Autodesk Inventor part; units mm, degrees
ref_plane "YZ Plane" through (0, 0, 0) normal (1, 0, 0) x (0, 1, 0)
ref_plane "XZ Plane" through (0, 0, 0) normal (0, 1, 0) x (-1, 0, 0)
ref_plane "XY Plane" through (0, 0, 0) normal (0, 0, 1) x (1, 0, 0)
sketch "Boceto1" plane through (0, 0, 0) normal (0, 1, 0) x (-1, 0, 0)
  line L0 (-10, 37.5) -> (10, 37.5)
  line L1 (10, 37.5) -> (10, -37.5)
  line L2 (10, -37.5) -> (-10, -37.5)
  line L3 (-10, -37.5) -> (-10, 37.5)
  line L4 (-10, 37.5) -> (10, -37.5) construction
  line L5 (10, 37.5) -> (-10, -37.5) construction
  circle A0 centre (0, -27.5) radius 8.125
  point P0 (0, 0)
  point P1 (5.4787, -34.25)
  point P2 (-5.4787, -34.25)
  dimension "d0" = 20
  dimension "d23" = 65
  dimension "d24" = 10
  dimension "d25" = 16.25
extrude "Extrusión1" add sketch "Boceto1" along normal blind 12 contours L0 L1 L2 L3 | A0
sketch "Boceto5" plane through (0, 12, 0) normal (0, 1, 0) x (1, 0, 0)
  circle A0 centre (0, 27.5) radius 8.125
  line L0 (10, 37.5) -> (-10, 37.5)
  line L1 (-10, -37.5) -> (10, -37.5)
  point P0 (0, 0)
  dimension "d26" = 16.25
  dimension "d36" = 65
extrude "Extrusión5" cut sketch "Boceto5" against normal blind 7
sketch "Boceto6" plane through (0, 5, -27.5) normal (0, 1, 0) x (1, 0, 0)
  circle A0 centre (0, 0) radius 6.5
  point P0 (0, -27.5)
  dimension "d30" = 13
extrude "Extrusión6" cut sketch "Boceto6" against normal through all
sketch "Boceto7" plane through (0, 12, 0) normal (0, 1, 0) x (1, 0, 0)
  circle A0 centre (0, 27.5) radius 8.125
  circle A1 centre (0, 27.5) radius 15
  point P0 (0, 0)
  dimension "d33" = 30
extrude "Extrusión7" cut sketch "Boceto7" against normal blind 2
fillet "Empalme5" radius 5 2 edges at (-10, 6, 37.5) (10, 6, 37.5)
fillet "Empalme6" radius 5 2 edges at (10, 5, -37.5) (-10, 5, -37.5)
sketch "Boceto8" plane through (0, 0, 0) normal (0, -1, 0) x (1, 0, 0)
  circle A0 centre (0, 31.5) radius 2.7
  circle A1 centre (0, 15.5) radius 2.7
  line L0 (-5, 37.5) -> (5, 37.5)
  circle A2 centre (0, -0.5) radius 2.7
  point P0 (0, 0)
  dimension "d39" = 5.4
  dimension "d40" = 6
  dimension "d41" = 16
  dimension "d47" = 16
extrude "Extrusión8" cut sketch "Boceto8" against normal through all
sketch "Boceto9" plane through (0, 0, 0) normal (0, -1, 0) x (1, 0, 0)
  circle A0 centre (0, 31.5) radius 2.7
  circle A1 centre (0, 31.5) radius 4.65
  circle A2 centre (0, 15.5) radius 2.7
  circle A3 centre (0, 15.5) radius 4.65
  circle A4 centre (0, -0.5) radius 2.7
  circle A5 centre (0, -0.5) radius 4.65
  point P0 (0, 0)
  dimension "d44" = 9.3
extrude "Extrusión9" cut sketch "Boceto9" against normal blind 2 contours A0 | A1 | A2 | A3 | A4 | A5
sketch "Boceto2" plane through (0, 12, 0) normal (0, 1, 0) x (1, 0, 0)
  line L0 (10, 37.5) -> (-10, 37.5)
  line L1 (-10, 37.5) -> (5, 37.5)
  line L2 (5, 37.5) -> (5, 77.5)
  line L3 (5, 77.5) -> (-5, 77.5)
  line L4 (-5, 77.5) -> (-5, 37.5)
  circle A0 centre (0, 70) radius 2.7
  line L5 (10, -37.5) -> (10, 37.5)
  line L6 (10, 37.5) -> (-10, 37.5)
  point P0 (0, 0)
  point P1 (5, 20)
  point P2 (-5, 20)
  dimension "d4" = 5.4
  dimension "d5" = 7.5
  dimension "d19" = 40
  dimension "d20" = 5
  dimension "d21" = 5
  dimension "d22" = 5
sketch "Boceto3" plane through (0, 10.5, 0) normal (0, -1, 0) x (1, 0, 0)
  circle A0 centre (0, -52.5) radius 2.7
  circle A1 centre (0, -52.5) radius 5
  line L0 (5, -60) -> (5, -20)
  point P0 (0, 0)
sketch "Boceto4" plane through (0, 0, 0) normal (0, -1, 0) x (1, 0, 0)
  circle A0 centre (0, -8) radius 2.7
  circle A1 centre (0, 8) radius 2.7
  point P0 (0, 0)
  dimension "d13" = 5.4
  dimension "d14" = 8
  dimension "d15" = 8
properties part number "top support"
CAD build for the part. Positions are in the model's coordinates, mm. A direction names the side the tool comes from. Coordinates: 2 decimals unless noted, no trailing zeros. Write each loop counter-clockwise with the first axis right and the second up, starting at its lowest first coordinate (ties: lowest second). Pieces come first, ordered by that corner, then holes. Notation, with made-up numbers: (-8, 54.5) - (0, 54.5) arc R22 cw to (0, 77.5) - close; hole circle Ø3 at (42, 19). An arc over 180 degrees is marked (long way). Use a Markdown table: item, result. Add a question column.
Item 1: Band-saw the part on A-A, the plane z = 15.5. Give the cut face in (x, y), and give its area (3 significant figures).
Item 2: Drill centre lines: L1, parallel to Z at x = 0, y = 1.55; L2, parallel to Z at x = 0, y = 2.1; L3, parallel to X at y = 8.5, z = -27.5 (3 decimals). Where is each one in solid material? Low to high. Write a range as from..to.
Item 3: Band-saw the part on D-D, the plane x = 0. Give the number of separate pieces and of enclosed holes in the cut face, and give its area (3 significant figures).
Item 4: Band-saw the part on C-C, the plane z = -27.5. Give the cut face in (x, y) (3 decimals).
Item 5: Mould opens along Z. For faces 1 (the face through (-0.351, 6.93, 18.177)), 2 (the face through (-8.57, 6.08, 36)), 3 (the face through (4, 10, -20)) say: pulls with the +Z half, pulls with the -Z half, needs draft (parallel to the pull), parting line crosses it, or undercut.
Item 6: Flat gauge pins, fed straight in: pin 1 (4.5 mm diameter, centred on x = 1, z = 0.5, fed in from -Y); pin 2 (6 mm diameter, centred on x = -3.5, z = -22, fed in from +Y); pin 3 (1.5 mm diameter, centred on x = -3.5, z = -21.5, fed in from +Y). Where does each tip first touch, or does it go through?
Item 7: 3-axis set-ups, long thin cutter, end or side, ignore diameter. For faces 4 (the face through (-4, 5, -33)), 5 (the face through (5, 0, 1)), 6 (the face through (2, 2, -3)), 7 (the face through (-10, 6, 0)), 8 (the face through (-0.2, 11, -12.5)): which of +Z, -Z, +X, -X, +Y, -Y reach the whole face in a straight line?
Item 8: Band-saw the part on B-B, the plane y = 9.25. Give the cut face in (x, z) (3 decimals), and give its area (3 significant figures).
Numbers:
| question | item | result |
|---|---|---|
| 1 | outline | (-10, 0) - (-4.65, 0) - (-4.65, 2) - (-2.7, 2) - (-2.7, 12) - (-10, 12) - close; (2.7, 2) - (4.65, 2) - (4.65, 0) - (10, 0) - (10, 12) - (2.7, 12) - close |
| 1 | area | 167 mm2 |
| 2 | L1 | -37.5..-34, -21..-5.15, 4.15..10.85, 20.15..26.85, 36.15..37.5 |
| 2 | L2 | -37.5..-34, -21..-3.2, 2.2..12.8, 18.2..28.8, 34.2..37.5 |
| 2 | L3 | -10..-8.125, 8.125..10 |
| 3 | separate pieces | 5 |
| 3 | enclosed holes | 0 |
| 3 | area | 486 mm2 |
| 4 | outline | (-10, 0) - (-6.5, 0) - (-6.5, 5) - (-8.125, 5) - (-8.125, 10) - (-10, 10) - close; (6.5, 0) - (10, 0) - (10, 10) - (8.125, 10) - (8.125, 5) - (6.5, 5) - close |
| 5 | face 1 | undercut |
| 5 | face 2 | pulls with the +Z half |
| 5 | face 3 | needs draft |
| 6 | pin 1 | y = 2 |
| 6 | pin 2 | y = 10 |
| 6 | pin 3 | y = 5 |
| 7 | face 4 | +Y |
| 7 | face 5 | +Z, -Z, +X, -X, -Y |
| 7 | face 6 | -Y |
| 7 | face 7 | +Z, -Z, -X, +Y, -Y |
| 7 | face 8 | -Z, +Y |
| 8 | outline | (-10, -32.5) arc R5 ccw to (-5, -37.5) - (5, -37.5) arc R5 ccw to (10, -32.5) - (10, 32.5) arc R5 ccw to (5, 37.5) - (-5, 37.5) arc R5 ccw to (-10, 32.5) - close; hole circle Ø16.25 at (0, -27.5); hole circle Ø5.4 at (0, -0.5); hole circle Ø5.4 at (0, 15.5); hole circle Ø5.4 at (0, 31.5) |
| 8 | area | 1,200 mm2 |
